Here's how the part is built. I have some questions about the finished solid (model axes, mm). A direction names the side the tool comes from. Round coordinates to 2 decimals unless told otherwise and drop trailing zeros. Loops run counter-clockwise (first coordinate to the right, second up) from the corner with the lowest first, then second, coordinate; pieces in that order, holes last. Notation, with made-up numbers: (60, -10) - (103, -10) arc R17 cw to (103, -2) - close; hole circle Ø3 at (82, 39). An arc over 180 degrees is marked (long way). Answer as a JSON object with one key per item and string values. Group by question number.
1) Will these pins go through, and if not, where does the flat tip stop? P1, Ø12, axis at x = -1, y = -9.5, coming from the -Z side; P2, Ø10, axis at x = -16, y = -20.5, coming from the +Z side.
2) If I drill on line 1 along Y through (x, z) = (31, 7.75); line 2 along X through (y, z) = (10, 12.75); line 3 along Z through (x, y) = (-9.5, -12), over which ranges is the centre line in solid material (lowest first)? Write a range as [from, to].
3) I want a section at C-C, the plane y = 4. Please give me the cut outline in (x, z), then the cut area to 3 significant figures.
4) I want a section at B-B, the plane x = 27.5. Please give me the cut outline in (y, z), then the cut area to 3 significant figures.
5) If we mould it in two halves opening along X, with no side actions, what happens to faces 1 (the face through (42.999, -9, 9)), 2 (the face through (9, -30.249, 9)), 3 (the face through (9, 11.151, 10))? For each: pulls with the +X half, pulls with the -X half, needs draft (parallel to the pull), parting line crosses it, or undercut.
6) Which directions (+Z, -Z, +X, -X, +Y, -Y) give clear straight access to the entire face, cutting with the end or side of a thin tool? Please do faces 4 (the face through (9, 12.151, 9)), 5 (the face through (-22.601, -9, 10)).
7) I want a section at A-A, the plane z = 9.75. Please give me the cut outline in (x, y), then the cut area to 3 significant figures.
from build123d import *

# Parameters (mm, degrees)
F0_W     = 66.6
F0_H     = 42.4
F1_DEPTH = 19
F2_T     = -1
F3_R     = 1.5
F4_DEPTH = 25
F5_R     = 1.5
F6_DEPTH = 25


with BuildPart() as f1:
    # F0 (on Top) → F1 (new body)
    with BuildSketch(Plane.XY):
        with Locations((9.69916, -9.049298)):
            Rectangle(F0_W, F0_H)
    extrude(amount=F1_DEPTH)

    # F2
    f2_openings = [f1.faces().sort_by_distance(p)[0] for p in [
        (9.69916, -9.049298, 19),
    ]]
    offset(amount=F2_T, openings=f2_openings)

    # F3 (on face) → F4 (cut)
    with BuildSketch(Plane(origin=(0, 0, 0), x_dir=(1, 0, 0), z_dir=(0, 0, -1))):
        with Locations((-11.35084, 25.999298)):
            Circle(F3_R)
    extrude(amount=-F4_DEPTH, mode=Mode.SUBTRACT)

    # F5 (on face) → F6 (cut)
    with BuildSketch(Plane(origin=(0, 0, 0), x_dir=(1, 0, 0), z_dir=(0, 0, -1))):
        with Locations((38.75916, -7.910702)):
            Circle(F5_R)
    extrude(amount=-F6_DEPTH, mode=Mode.SUBTRACT)


solid = f1.part
Outcome:
{
 "1": {"P1": "z = 0", "P2": "z = 1"},
 "2": {"line 1": "[-30.25, -29.25], [11.15, 12.15]", "line 2": "[-23.6, -22.6], [42, 43]", "line 3": "[0, 1]"},
 "3": {"outline": "(-23.6, 0) - (43, 0) - (43, 19) - (42, 19) - (42, 1) - (-22.6, 1) - (-22.6, 19) - (-23.6, 19) - close", "area": "103 mm^2"},
 "4": {"outline": "(-30.25, 0) - (12.15, 0) - (12.15, 19) - (11.15, 19) - (11.15, 1) - (-29.25, 1) - (-29.25, 19) - (-30.25, 19) - close", "area": "78.4 mm^2"},
 "5": {"face 1": "pulls with the +X half", "face 2": "needs draft", "face 3": "undercut"},
 "6": {"face 4": "+Z, -Z, +X, -X, +Y", "face 5": "+Z"},
 "7": {"outline": "(-23.6, -30.25) - (43, -30.25) - (43, 12.15) - (-23.6, 12.15) - close; hole (-22.6, -29.25) - (42, -29.25) - (42, 11.15) - (-22.6, 11.15) - close", "area": "214 mm^2"}
}
